Model file for the job. Use its own axes, mm. A direction names the side the tool comes from. Round coordinates to 2 decimals unless told otherwise and drop trailing zeros. Order: outer loops, then holes, each group sorted by start corner. A loop starts at its lowest first (then second) coordinate and runs counter-clockwise, first axis right, second up. Notation, with made-up numbers: (32.5, -35.75) - (64.5, -35.75) arc R23 ccw to (64.5, -23.75) - close; hole circle Ø10 at (45.5, 53). An arc over 180 degrees is marked (long way). Write item = value, one per line.
```python
from build123d import *

# Parameters (mm, degrees)
SCHIZZO1_W                   = 16.07
SCHIZZO1_H                   = 14.64
ESTRUSIONE_ESTRUSIONE1_DEPTH = 1.96
TAGLIO_ESTRUSIONE1_DEPTH     = 12.044692164
SCHIZZO3_R                   = 1.5
TAGLIO_ESTRUSIONE2_DEPTH     = 12.044692164


with BuildPart() as part:
    # Schizzo1 → Estrusione-Estrusione1 (new body)
    with BuildSketch(Plane.XY):
        Rectangle(SCHIZZO1_W, SCHIZZO1_H)
    extrude(amount=-ESTRUSIONE_ESTRUSIONE1_DEPTH)

    # Schizzo2 → Taglio-Estrusione1 (cut, through all)
    with BuildSketch(Plane.XY):
        Polygon((-4.78, 0.18), (-4.78, 7.32), (-8.035, 7.32), (-8.035, -2.12), align=None)
        Polygon((8.035, 7.32), (4.78, 7.32), (4.78, 0.18), (8.035, -2.12), align=None)
    extrude(amount=-TAGLIO_ESTRUSIONE1_DEPTH, mode=Mode.SUBTRACT)

    # Schizzo3 → Taglio-Estrusione2 (cut, through all)
    with BuildSketch(Plane.XY):
        with Locations((-5, -4.67)):
            Circle(SCHIZZO3_R)
        with Locations((5, -4.67)):
            Circle(SCHIZZO3_R)
    extrude(amount=-TAGLIO_ESTRUSIONE2_DEPTH, mode=Mode.SUBTRACT)


solid = part.part
```
1) 3-axis set-ups, long thin cutter, end or side, ignore diameter. For faces 1 (the face through (4.78, 4, -1)), 2 (the face through (-4.78, 4, -1)), 3 (the face through (0, -2, 0)): which of +Z, -Z, +X, -X, +Y, -Y reach the whole face in a straight line?
Conclusion:
face_1 = +Z, -Z, +X, +Y
face_2 = +Z, -Z, -X, +Y
face_3 = +Z, +X, -X, +Y, -Y
2) Cut at D-D (y = 1.75). Write the cut outline in (x, z).
Conclusion:
outline = (-4.78, -1.96) - (4.78, -1.96) - (4.78, 0) - (-4.78, 0) - close
3) Cut at B-B (z = -1.2). Write the cut outline in (x, y) (3 decimals).
Conclusion:
outline = (-8.035, -7.32) - (8.035, -7.32) - (8.035, -2.12) - (4.78, 0.18) - (4.78, 7.32) - (-4.78, 7.32) - (-4.78, 0.18) - (-8.035, -2.12) - close; hole circle Ø3 at (-5, -4.67); hole circle Ø3 at (5, -4.67)
4) Cut at A-A (y = -4.67). Write the cut outline in (x, z) (3 decimals).
Conclusion:
outline = (-8.035, -1.96) - (-6.5, -1.96) - (-6.5, 0) - (-8.035, 0) - close; (-3.5, -1.96) - (3.5, -1.96) - (3.5, 0) - (-3.5, 0) - close; (6.5, -1.96) - (8.035, -1.96) - (8.035, 0) - (6.5, 0) - close
5) Mould opens along Y. For faces 4 (the face through (6.386, -5.245, -0.966)), 5 (the face through (-8.035, -5, -1)), 6 (the face through (0, 7.32, -1)) say: +Y half, -Y half, draft (parallel to the pull), parting line (faces both ways), or undercut.
Conclusion:
face_4 = undercut
face_5 = draft
face_6 = +Y half
6) Wall check: line 1 along X through (y, z) = (-6, -1.1) (3 decimals); line 2 along X through (y, z) = (4.25, -1.15); line 3 along Y through (x, z) = (-5.75, -1.8). Give the ranges that are in metal, low to high.
Conclusion:
line_1 = -8.035 to -5.694, -4.306 to 4.306, 5.694 to 8.035
line_2 = -4.78 to 4.78
line_3 = -7.32 to -5.97, -3.37 to -0.51
7) Cut at C-C (x = -5.5). Write the cut outline in (y, z).
Conclusion:
outline = (-7.32, -1.96) - (-6.08, -1.96) - (-6.08, 0) - (-7.32, 0) - close; (-3.26, -1.96) - (-0.33, -1.96) - (-0.33, 0) - (-3.26, 0) - close
